Geometry: see drawing. Coordinates: mm, zero at the bounding-box minimum. A direction names the side the tool comes from. Round coordinates to 2 decimals unless told otherwise and drop trailing zeros. Order: outer loops, then holes, each group sorted by start corner. A loop starts at its lowest first (then second) coordinate and runs counter-clockwise, first axis right, second up. Notation, with made-up numbers: (-11, 23) -> (-6, 23) arc R22 ccw to (-6, 33) -> close; hole circle Ø6 at (-10.5, -26.5). An arc over 180 degrees is marked (long way). Answer as CSV lines item,"result". Start each with the question number.
(1) Set-up query: the marked faces 1, 2 and 3. Return all of +Z, -Z, +X, -X, +Y, -Y with unobstructed straight access to the full face (end or side cutting, diameter ignored); none if empty.
(2) Pull-direction query (Y, two-part tool) for the marked faces 4, 5 and 6; classes: +Y half, -Y half, draft (parallel to the pull), parting line (faces both ways), or undercut.
(3) Section query A-A (y = 28.25). Output: boundary loops of the cut face in (x, z), plus the area to 3 significant figures.
(4) Section query B-B (y = 10.5). Output: boundary loops of the cut face in (x, z), plus the area to 3 significant figures.
(5) Line query: line 1 along Z through (x, y) = (8, 13.25); line 2 along Y through (x, z) = (18, 16); line 3 along Y through (x, z) = (19.25, 5) (1 decimal). Output: solid intervals per line, ascending. Write a range as from..to.
(6) Contact query for flat-ended pins moving along their axis: P1, Ø4, axis at x = 9.5, y = 27, coming from the -Z side; P2, Ø3, axis at x = 7.5, y = 27.5, coming from the +Z side; P3, Ø6, axis at y = 8, z = 3, coming from the -X side. Output: stop coordinate, or through.
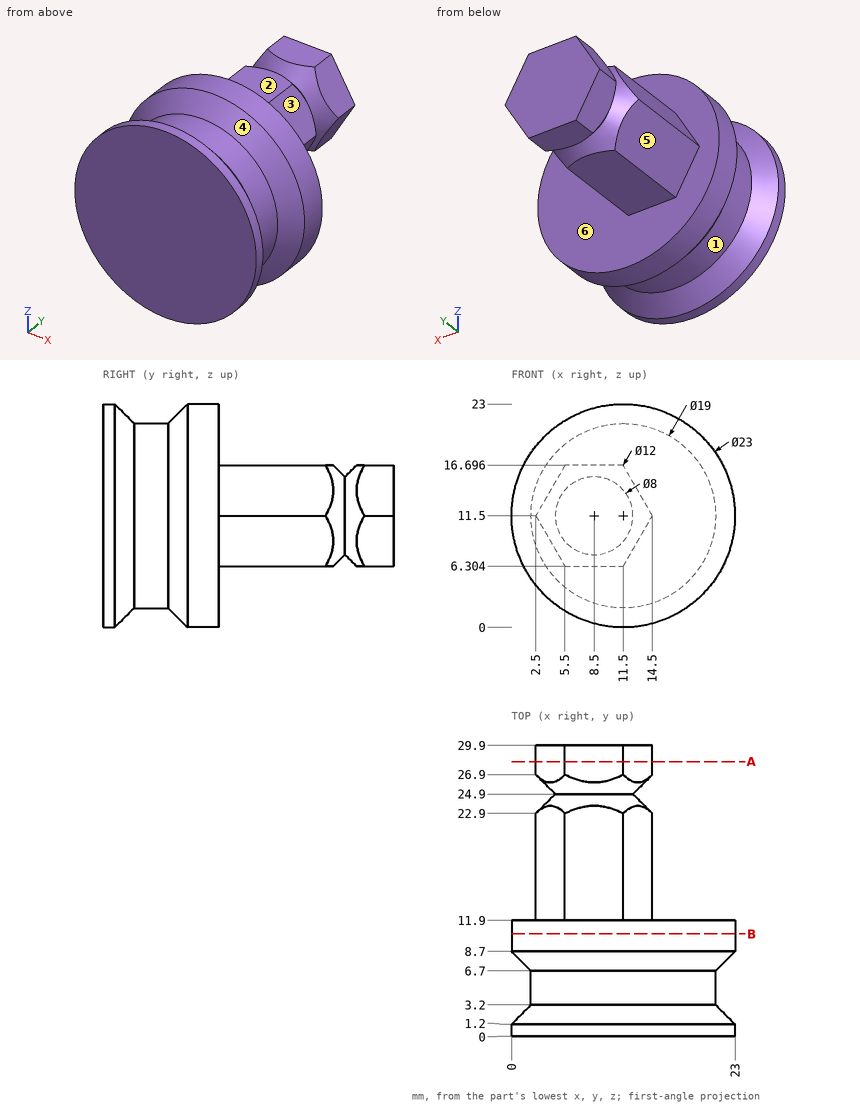
Answer block:
1,face 1,"none"
1,face 2,"+Z, +X, -X, +Y"
1,face 3,"+Z, +X, +Y"
2,face 4,"undercut"
2,face 5,"draft"
2,face 6,"+Y half"
3,outline,"(2.5, 11.5) -> (5.5, 6.3) -> (11.5, 6.3) -> (14.5, 11.5) -> (11.5, 16.7) -> (5.5, 16.7) -> close"
3,area,"93.5 mm2"
4,outline,"circle Ø23 at (11.5, 11.5)"
4,area,"415 mm2"
5,line 1,"6.3..16.7"
5,line 2,"0..11.9"
5,line 3,"0..2.6, 7.3..11.9"
6,P1,"z = 6.3"
6,P2,"z = 16.7"
6,P3,"x = 1.45"
